Autodesk Fusion 360 part; units mm, degrees
sketch "Sketch1" plane through (0, 0, 0) normal (0, 0, 1) x (1, 0, 0)
  line L0 (-25, 25) -> (25, 25)
  line L1 (25, 25) -> (25, -25)
  line L2 (25, -25) -> (-25, -25)
  line L3 (-25, -25) -> (-25, 25)
  dimension "d1" = 25
  dimension "d2" = 25
  dimension "d3" = 25
  dimension "d4" = 25
extrude "Extrude1" add sketch "Sketch1" along normal blind 1.6
equation "d2 = d1"
equation "d3 = d1"
equation "d4 = d1"

Autodesk Fusion 360 part; units mm, degrees
sketch "Sketch1" plane through (0, 0, 0) normal (0, 0, 1) x (1, 0, 0)
  line L0 (90, 95) -> (-90, 95)
  line L1 (-95, 90) -> (-95, -90)
  line L2 (-90, -95) -> (90, -95)
  line L3 (95, -90) -> (95, 90)
  arc A0 (95, 90) -> (90, 95) centre (90, 90) ccw
  arc A1 (-90, 95) -> (-95, 90) centre (-90, 90) ccw
  arc A2 (-95, -90) -> (-90, -95) centre (-90, -90) ccw
  arc A3 (90, -95) -> (95, -90) centre (90, -90) ccw
  point P0 (95, 95)
  point P1 (-95, 95)
  point P2 (95, -95)
  dimension "d1" = 190
  dimension "d2" = 190
  dimension "d3" = 95
  dimension "d4" = 95
  dimension "d5" = 5
extrude "Extrude1" add sketch "Sketch1" along normal blind 5
sketch "Sketch2" plane through (0, 0, 0) normal (0, 0, -1) x (1, 0, 0)
  arc A0 (95, 90) -> (90, 95) centre (90, 90) ccw
  line L0 (90, 95) -> (-90, 95)
  arc A1 (-90, 95) -> (-95, 90) centre (-90, 90) ccw
  line L1 (-95, 90) -> (-95, -90)
  arc A2 (-95, -90) -> (-90, -95) centre (-90, -90) ccw
  line L2 (-90, -95) -> (90, -95)
  arc A3 (90, -95) -> (95, -90) centre (90, -90) ccw
  line L3 (95, -90) -> (95, 90)
  line L4 (-95, 95) -> (95, 95)
  line L5 (95, 95) -> (95, -95)
  line L6 (95, -95) -> (-95, -95)
  line L7 (-95, -95) -> (-95, 95)
  line L8 (95, -95) -> (75, -95)
  line L9 (75, -95) -> (75, -75)
  line L10 (75, -75) -> (95, -75)
  line L11 (95, -75) -> (95, -95)
  line L12 (-95, -95) -> (-75, -95)
  line L13 (-75, -95) -> (-75, -75)
  line L14 (-75, -75) -> (-95, -75)
  line L15 (-95, -75) -> (-95, -95)
  line L16 (95, 95) -> (75, 95)
  line L17 (75, 95) -> (75, 75)
  line L18 (75, 75) -> (95, 75)
  line L19 (95, 75) -> (95, 95)
  line L20 (-95, 95) -> (-75, 95)
  line L21 (-75, 95) -> (-75, 75)
  line L22 (-75, 75) -> (-95, 75)
  line L23 (-95, 75) -> (-95, 95)
  dimension "d8" = 20
  dimension "d9" = 20
extrude "Extrude2" add sketch "Sketch2" along normal blind 5 contours L0 L1 L2 L3 L4 L5 L6 L7 L9 L10 L13 L14 L17 L18 L21 L22
equation "d2 = d1"
equation "d3 = d1 / 2"
equation "d4 = d1 / 2"
Input: part model. Units: mm. Frame: model coordinates. A direction names the side the tool comes from. Coordinates: 2 decimals unless noted, no trailing zeros. Order: outer loops, then holes, each group sorted by start corner. A loop starts at its lowest first (then second) coordinate and runs counter-clockwise, first axis right, second up. Notation, with made-up numbers: M 49,-33 L 60,-33 A26 cw 60,-15 Z; hole C -37,66 d11. An arc over 180 degrees is marked long. Answer in a Markdown table with one row per item.
(1) Contact query for flat-ended pins moving along their axis: pin 1 Ø10 at (x, y) = (-88.5, 87) entering from -Z; pin 2 Ø1.5 at (y, z) = (85, -2) entering from +X; pin 3 Ø1.5 at (x, z) = (84.5, -2.5) entering from -Y. Output: stop coordinate, or through.
Numbers:
| item | result |
|---|---|
| pin 1 | stops at z = 0 |
| pin 2 | stops at x = 75 |
| pin 3 | stops at y = -75 |
(2) Section query A-A, the plane z = -2. Output: boundary loops of the cut face in (x, y).
Numbers:
| item | result |
|---|---|
| outline | M -95,-75 L -75,-75 L -75,-95 L 75,-95 L 75,-75 L 95,-75 L 95,75 L 75,75 L 75,95 L -75,95 L -75,75 L -95,75 Z |
(3) Access query for faces 1 (the flat face through (75, 85, -2)), 2 (the flat face through (75, -85, -2)), 3 (the flat face through (-85, -75, -2)), 4 (the flat face through (-85, 85, 0)). Directions: +Z, -Z, +X, -X, +Y, -Y. A direction counts if a zero-diameter tool reaches every point of the face in a straight line with its end or side. Return the directions, or none.
Numbers:
| item | result |
|---|---|
| face 1 | -Z, +X, +Y |
| face 2 | -Z, +X, -Y |
| face 3 | -Z, -X, -Y |
| face 4 | -Z, -X, +Y |
(4) Material intervals for line 1 (Y direction, x = 83, z = -2), sorted ascending. Write a range as [from, to].
Numbers:
| item | result |
|---|---|
| line 1 | y = [-75, 75] |
